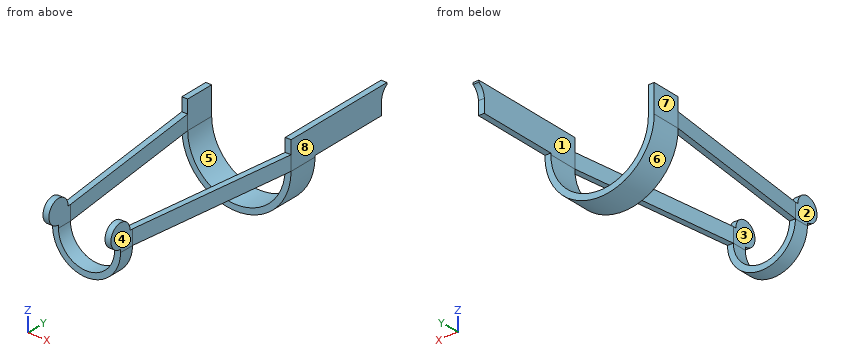
from build123d import *

# Parameters (mm, degrees)
EXTRUDE_1_DEPTH     = 20
SKETCH_3_R          = 16
EXTRUDE_2_DEPTH     = 8
EXTRUDE_START       = -8
SKETCH_4_R          = 16
EXTRUDE_3_DEPTH     = 8
EXTRUDE_4_DEPTH     = 20
SKETCH_5_W          = 8
SKETCH_5_H          = 20
SKETCH_7_W          = 8
SKETCH_7_H          = 20
SKETCH_10_W         = 8
SKETCH_10_H         = 36
EXTRUDE_5_DEPTH     = 160
CUT_EXTRUDE_3_DEPTH = 160
SKETCH_13_W         = 62.199259601
SKETCH_13_H         = 136.537597085
CUT_EXTRUDE_4_DEPTH = 10


with BuildPart() as part:
    # Sketch 2 → Extrude 1 (new body)
    with BuildSketch(Plane(origin=(0, 0, 0), x_dir=(1, 0, 0), z_dir=(0, 1, 0))):
        with BuildLine():
            Line((-46, 0), (-46, -20))
            Line((-46, -20), (-38, -20))
            Line((-38, -20), (-38, 0))
            ThreePointArc((-38, 0), (0, 38), (38, 0))
            Line((38, 0), (38, -20))
            Line((38, -20), (46, -20))
            Line((46, -20), (46, 0))
            ThreePointArc((46, 0), (0, 46), (-46, 0))
        make_face()
    extrude(amount=EXTRUDE_1_DEPTH)

    # Sketch 3 → Extrude 2 (add)
    with BuildSketch(Plane.ZY.offset(46)):
        with Locations((20, 0)):
            Circle(SKETCH_3_R)
    extrude(amount=-EXTRUDE_2_DEPTH)

    # Sketch 4 → Extrude 3 (add)
    with BuildSketch(Plane(origin=(46, 0, 0), x_dir=(0, 0, -1), z_dir=(1, 0, 0)).offset(EXTRUDE_START)):
        with Locations((-20, 0)):
            Circle(SKETCH_4_R)
    extrude(amount=EXTRUDE_3_DEPTH)



with BuildPart() as body_2:
    # Sketch 3D_1 → Extrude 4 (new, symmetric)
    with BuildSketch(Plane(origin=(-74, 270, 0), x_dir=(0.9909924304103234, 0, 0.13391789600139506), z_dir=(0, -1, 0))):
        with BuildLine():
            Line((0, 0), (2.67835792, 19.819848608))
            Line((2.67835792, 19.819848608), (10.606297363, 18.74850544))
            Line((10.606297363, 18.74850544), (7.927939443, -1.071343168))
            ThreePointArc((7.927939443, -1.071343168), (64.494858714, -75.315424711), (138.738940257, -18.74850544))
            Line((138.738940257, -18.74850544), (141.417298177, 1.071343168))
            Line((141.417298177, 1.071343168), (149.345237621, 0))
            Line((149.345237621, 0), (146.666879701, -19.819848608))
            ThreePointArc((146.666879701, -19.819848608), (63.423515546, -83.243364154), (0, 0))
        make_face()
    extrude(amount=EXTRUDE_4_DEPTH, both=True)


with BuildPart() as part_1:
    add(part.part)

    add(body_2.part)  # Sweep 1 merges body 2
    # Sweep 1: sweep along a path in Sketch 6
    with BuildLine(Plane.XY.offset(20)) as sweep_1_path:
        Line((46, 20), (74, 250))
    # Sketch 5 → Sweep 1 (sweep)
    with BuildSketch(Plane(origin=(0, 20, 0), x_dir=(1, 0, 0), z_dir=(0, 1, 0))):
        with Locations((42, -10)):
            Rectangle(SKETCH_5_W, SKETCH_5_H)
    sweep(path=sweep_1_path.line)

    # Sweep 2: sweep along a path in Sketch 8
    with BuildLine(Plane.XY.offset(20)) as sweep_2_path:
        Line((-46, 20), (-74, 250))
    # Sketch 7 → Sweep 2 (sweep)
    with BuildSketch(Plane(origin=(0, 20, 0), x_dir=(1, 0, 0), z_dir=(0, 1, 0))):
        with Locations((-42, -10)):
            Rectangle(SKETCH_7_W, SKETCH_7_H)
    sweep(path=sweep_2_path.line)

    # Sketch 10 → Extrude 5 (add)
    with BuildSketch(Plane.XZ.offset(-250)):
        with Locations((-70, 20)):
            Rectangle(SKETCH_10_W, SKETCH_10_H)
        with Locations((70, 20)):
            Rectangle(SKETCH_10_W, SKETCH_10_H)
    extrude(amount=-EXTRUDE_5_DEPTH)

    # Sketch 12 → Cut-Extrude 3 (cut)
    with BuildSketch(Plane.ZY.offset(74)):
        with BuildLine():
            Line((20, 401), (2, 401))
            Line((2, 401), (2, 419))
            ThreePointArc((2, 419), (32.727922061, 431.727922061), (20, 401))
        make_face()
    extrude(amount=-CUT_EXTRUDE_3_DEPTH, mode=Mode.SUBTRACT)

    # Sketch 13 → Cut-Extrude 4 (cut)
    with BuildSketch(Plane.ZY.offset(74)):
        with Locations((25.303398621, 358.268798543)):
            Rectangle(SKETCH_13_W, SKETCH_13_H)
    extrude(amount=-CUT_EXTRUDE_4_DEPTH, mode=Mode.SUBTRACT)


solid = part_1.part
Geometry check sheet. Reference: the model listing, model coordinates, mm. Face numbers are marked on the shaded views. A direction names the side the tool comes from. Round coordinates to 2 decimals unless told otherwise and drop trailing zeros. Order: outer loops, then holes, each group sorted by start corner. A loop starts at its lowest first (then second) coordinate and runs counter-clockwise, first axis right, second up. Notation, with made-up numbers: M 26.25,88.5 L 84.25,88.5 A34 ccw 84.25,120.5 Z; hole C 0.25,15.25 d3. An arc over 180 degrees is marked long. Write each question's results on one line, items separated by ' | '. Start each with the question number.
1. Go/stop test with flat-tipped pins: P1, Ø2, axis at y = 211, z = 11, coming from the +X side; P2, Ø11, axis at x = 61, y = 158, coming from the -Z side; P3, Ø1.5, axis at x = -38.5, y = 44.5, coming from the +Z side; P4, Ø11, axis at x = 61.5, y = 137.5, coming from the +Z side. Record where each tip stops, or that it passes through.
2. Set-up check for the marked faces 1, 2, 3 and 4: record each of +Z, -Z, +X, -X, +Y, -Y from which the full face is reachable in a straight line by a thin tool's end or side.
3. Draft check along X on the marked faces 5, 6, 7 and 8. Enter one of: pulls with the +X half, pulls with the -X half, needs draft (parallel to the pull), parting line crosses it, or undercut.
4. Cross-section at B-B on y = 29. Record the boundary of the cut face in (x, z), plus the area to 3 significant figures.
5. Cross-section at C-C on y = 350.5. Record the boundary of the cut face in (x, z).
6. Cross-section at A-A on x = 0. Record the boundary of the cut face in (y, z), plus the area to 3 significant figures.
7. Material ranges on L1, parallel to X at y = 260.5, z = 30.5; L2, parallel to X at y = 25, z = 18.5; L3, parallel to Z at x = -63.5, y = 205, recorded low to high. Write a range as from..to.
Resolved:
1) P1: x = 69.37 | P2: z = 0 | P3: through | P4: z = 20
2) face 1: +Z, +Y | face 2: +Z, -Z, -X, -Y | face 3: +Z, +Y, -Y | face 4: +Z, -Z, +X, -Y
3) face 5: undercut | face 6: parting line crosses it | face 7: pulls with the -X half | face 8: pulls with the +X half
4) outline: M -47.1,0 L -39.1,0 L -39.1,20 L -47.1,20 Z; M 39.1,0 L 47.1,0 L 47.1,20 L 39.1,20 Z | area: 320 mm2
5) outline: M 66,2 L 74,2 L 74,38 L 66,38 Z
6) outline: M 0,-46 L 20,-46 L 20,-38 L 0,-38 Z; M 250,-74 L 290,-74 L 290,-66 L 250,-66 Z | area: 480 mm2
7) L1: -74..-66, 66..74 | L2: -46.61..-38.61, 38.61..46.61 | L3: 0..20
